Source: CAD feature listing. Evaluate the final solid. Frame: model axes, mm. A direction names the side the tool comes from. Give positions to 0.01 mm unless a question says otherwise; leave off trailing zeros. Order: outer loops, then holes, each group sorted by start corner. A loop starts at its lowest first (then second) coordinate and runs counter-clockwise, first axis right, second up. Notation, with made-up numbers: M -31.75,55.5 L 12.25,55.5 A14 ccw 12.25,77.5 Z; hole C 28,22.5 d9. An arc over 180 degrees is marked long. Return JSON: item names as keys, results as strings.
from build123d import *

# Parameters (mm, degrees)
BOSS_EXTRUDE1_DEPTH = 9
SKETCH2_R           = 0.5
CUT_EXTRUDE1_DEPTH  = 9
BOSS_EXTRUDE2_DEPTH = 0.5


with BuildPart() as part:
    # Sketch1 → Boss-Extrude1 (new body)
    with BuildSketch(Plane(origin=(0, 0, 0), x_dir=(1, 0, 0), z_dir=(0, 1, 0))):
        with BuildLine():
            Line((12.508, 0), (14.291457286, 0))
            Line((14.291457286, 0), (16, 0))
            Line((16, 0), (16, 1))
            Line((16, 1), (13.508, 1))
            Line((13.508, 1), (13, 1))
            Line((13, 1), (13, 1.508))
            Line((13, 1.508), (13, 10.492))
            ThreePointArc((13, 10.492), (12.851210245, 10.851210245), (12.492, 11))
            Line((12.492, 11), (-0.492, 11))
            ThreePointArc((-0.492, 11), (-0.851210245, 10.851210245), (-1, 10.492))
            Line((-1, 10.492), (-1, 1.508))
            Line((-1, 1.508), (-1, 1))
            Line((-1, 1), (-1.508, 1))
            Line((-1.508, 1), (-4, 1))
            Line((-4, 1), (-4, 0))
            Line((-4, 0), (-0.904522613, 0))
            Line((-0.904522613, 0), (-0.508, 0))
            Line((-0.508, 0), (0, 0))
            Line((0, 0), (0, 0.508))
            Line((0, 0.508), (0, 9.492))
            ThreePointArc((0, 9.492), (0.148789755, 9.851210245), (0.508, 10))
            Line((0.508, 10), (11.492, 10))
            ThreePointArc((11.492, 10), (11.851210245, 9.851210245), (12, 9.492))
            Line((12, 9.492), (12, 0.508))
            Line((12, 0.508), (12, 0))
            Line((12, 0), (12.508, 0))
        make_face()
    extrude(amount=BOSS_EXTRUDE1_DEPTH)

    # Sketch2 → Cut-Extrude1 (cut)
    with BuildSketch(Plane(origin=(0, 0, -1), x_dir=(-1, 0, 0), z_dir=(0, 0, -1))):
        with Locations((3, 1)):
            Circle(SKETCH2_R)
        with Locations((3, 8)):
            Circle(SKETCH2_R)
        with Locations((-15, 1)):
            Circle(SKETCH2_R)
        with Locations((-15, 8)):
            Circle(SKETCH2_R)
    extrude(amount=-CUT_EXTRUDE1_DEPTH, mode=Mode.SUBTRACT)

    # Sketch3 → Boss-Extrude2 (add)
    with BuildSketch(Plane(origin=(0, 4.50000011, 0), x_dir=(1, 0, 0), z_dir=(0, 1, 0))):
        Polygon((-3, 1), (-1, 8), (-1, 1), align=None)
        Polygon((13, 8), (13, 1), (15, 1), align=None)
    extrude(amount=BOSS_EXTRUDE2_DEPTH)


solid = part.part
1. Section query C-C (y = 3). Return loops of the section in (x, z), then the cut area to 3 significant figures.
Evaluation:
{"outline": "M -4,-1 L -1,-1 L -1,-10.49 A0.51 ccw -0.49,-11 L 12.49,-11 A0.51 ccw 13,-10.49 L 13,-1 L 16,-1 L 16,0 L 12,0 L 12,-9.49 A0.51 cw 11.49,-10 L 0.51,-10 A0.51 cw 0,-9.49 L 0,0 L -4,0 Z", "area": "40.0 mm^2"}
2. Section query B-B (z = -5.5). Return loops of the section in (x, y), then the cut area to 3 significant figures.
Evaluation:
{"outline": "M -1.71,4.5 L -1,4.5 L -1,0 L 0,0 L 0,9 L -1,9 L -1,5 L -1.71,5 Z; M 12,0 L 13,0 L 13,4.5 L 13.71,4.5 L 13.71,5 L 13,5 L 13,9 L 12,9 Z", "area": "18.7 mm^2"}
3. First-contact query: pin 1 (1.6 mm diameter, centred on x = 14, z = -4.5, fed in from -Y); pin 2 (2 mm diameter, centred on y = 3.5, z = -8.5, fed in from +X); pin 3 (1 mm diameter, centred on x = 14, z = -3, fed in from +Y). Flat tips, straight axial feed; report the tip coordinate or a pass-through.
Evaluation:
{"pin 1": "stops at y = 4.5", "pin 2": "stops at x = 13", "pin 3": "stops at y = 5"}
4. Ray query, probe 1 along Y at (x, z) = (15, -0.25); probe 2 along X at (y, z) = (6.25, -7.25); probe 3 along Z at (x, y) = (13.5, 7.75). Return the intervals inside material, ascending.
Evaluation:
{"probe 1": "y = 0 to 0.5, 1.5 to 7.5, 8.5 to 9", "probe 2": "x = -1 to 0, 12 to 13", "probe 3": "z = -1 to 0"}
5. Section query D-D (y = 8.25). Return loops of the section in (x, z), then the cut area to 3 significant figures.
Evaluation:
{"outline": "M -4,-1 L -3.43,-1 L -3.43,0 L -4,0 Z; M -2.57,-1 L -1,-1 L -1,-10.49 A0.51 ccw -0.49,-11 L 12.49,-11 A0.51 ccw 13,-10.49 L 13,-1 L 14.57,-1 L 14.57,0 L 12,0 L 12,-9.49 A0.51 cw 11.49,-10 L 0.51,-10 A0.51 cw 0,-9.49 L 0,0 L -2.57,0 Z; M 15.43,-1 L 16,-1 L 16,0 L 15.43,0 Z", "area": "38.3 mm^2"}
6. Draft query along X for faces 5 (the face through (14, 4, 0)), 6 (the face through (-1, 4, -6)), 7 (the face through (12, 4, -5)). Return one class per face: pulls with the +X half, pulls with the -X half, needs draft (parallel to the pull), parting line crosses it, or undercut.
Evaluation:
{"face 5": "needs draft", "face 6": "pulls with the -X half", "face 7": "undercut"}
7. Set-up query: faces 1 (the face through (14, 5, -3)), 2 (the face through (-2, 4, -1)), 3 (the face through (0, 4, -5)), 4 (the face through (13, 4, -6)). Return all of +Z, -Z, +X, -X, +Y, -Y with unobstructed straight access to the full face (end or side cutting, diameter ignored); none if empty.
Evaluation:
{"face 1": "-Z, +X, +Y", "face 2": "-Z, -X", "face 3": "+Z, +Y, -Y", "face 4": "-Z, +X"}
8. Section query A-A (y = 1). Return loops of the section in (x, z).
Evaluation:
{"outline": "M -4,-1 L -3.5,-1 L -3.5,0 L -4,0 Z; M -2.5,-1 L -1,-1 L -1,-10.49 A0.51 ccw -0.49,-11 L 12.49,-11 A0.51 ccw 13,-10.49 L 13,-1 L 14.5,-1 L 14.5,0 L 12,0 L 12,-9.49 A0.51 cw 11.49,-10 L 0.51,-10 A0.51 cw 0,-9.49 L 0,0 L -2.5,0 Z; M 15.5,-1 L 16,-1 L 16,0 L 15.5,0 Z"}
